from build123d import *

# Parameters (mm, degrees)
MODEL_R             = 2
MODEL_R_2           = 1.5
BOSS_EXTRUDE1_DEPTH = 6


with BuildPart() as part:
    # Model → Boss-Extrude1 (new body)
    with BuildSketch(Plane.XY):
        Polygon((136.503533409, 63.253129949), (136.50298126, 57.754435229), (123.504343338, 57.752522637), (123.503533606, 63.255740591), (110.504895018, 63.258351095), (110.504341961, 57.750609844), (97.50570415, 57.760961628), (97.504895084, 63.259656484), (84.506256496, 63.262266989), (84.505704216, 57.762267017), (71.507065628, 57.764877521), (71.508169139, 63.259656429), (71.52323132, 218.754434691), (84.52187017, 218.754434691), (84.52131789, 213.254434719), (97.51995674, 213.254434719), (97.521870105, 218.753129302), (110.520509732, 218.760870582), (110.519956675, 213.25312933), (123.518595525, 213.25312933), (123.520510463, 218.75634701), (136.519147739, 218.751823913), (136.51859559, 213.253129193), (149.517234309, 213.251823941), (149.512489722, 166.001824179), (143.512489752, 166.002426666), (143.512213612, 163.25242668), (143.511937472, 160.502426694), (149.511937442, 160.501824207), (149.50867397, 128.001824371), (143.508674, 128.002426858), (143.50839786, 125.252426872), (143.50812172, 122.502426886), (149.502172128, 122.501824996), (149.502172128, 63.251824697), align=None)
        with Locations((110.507816209, 83.257045523)):
            Circle(MODEL_R, mode=Mode.SUBTRACT)
        with Locations((110.518861547, 193.254434719)):
            Circle(MODEL_R, mode=Mode.SUBTRACT)
        with Locations((110.507264687, 138.255740731)):
            Circle(MODEL_R_2, mode=Mode.SUBTRACT)
        Polygon((119.512213733, 163.254836629), (119.512489873, 166.004836615), (125.512489843, 166.004234128), (125.511937563, 160.504234156), (119.511937593, 160.504836643), align=None, mode=Mode.SUBTRACT)
        Polygon((131.512213673, 163.253631655), (131.512489813, 166.003631641), (137.512489783, 166.003029154), (137.511937503, 160.503029181), (131.511937533, 160.503631669), align=None, mode=Mode.SUBTRACT)
        Polygon((113.511008789, 151.255439177), (113.511284929, 154.005439163), (119.511284899, 154.004836676), (119.510732619, 148.504836703), (113.510732649, 148.505439191), align=None, mode=Mode.SUBTRACT)
        Polygon((125.511008729, 151.254234202), (125.511284869, 154.004234189), (131.511284838, 154.003631701), (131.510732558, 148.503631729), (125.510732589, 148.504234216), align=None, mode=Mode.SUBTRACT)
        Polygon((137.511008668, 151.253029228), (137.511284808, 154.003029214), (143.511284778, 154.002426727), (143.510732498, 148.502426755), (137.510732528, 148.503029242), align=None, mode=Mode.SUBTRACT)
        Polygon((119.508397981, 125.254836821), (119.508674121, 128.004836807), (125.508674091, 128.00423432), (125.508121811, 122.504234347), (119.508121841, 122.504836835), align=None, mode=Mode.SUBTRACT)
        Polygon((131.50839792, 125.253631846), (131.50867406, 128.003631832), (137.50867403, 128.003029345), (137.50812175, 122.503029373), (131.50812178, 122.50363186), align=None, mode=Mode.SUBTRACT)
        Polygon((125.507192976, 113.254234394), (125.507469116, 116.00423438), (131.507469086, 116.003631893), (131.506916806, 110.503631921), (125.506916836, 110.504234408), align=None, mode=Mode.SUBTRACT)
        Polygon((137.507192916, 113.253029419), (137.507469056, 116.003029406), (143.507469025, 116.002426918), (143.506916745, 110.502426946), (137.506916776, 110.503029433), align=None, mode=Mode.SUBTRACT)
    extrude(amount=BOSS_EXTRUDE1_DEPTH)


solid = part.part
Build history of the part. All positions in model axes, mm. Round coordinates to 2 decimals unless told otherwise and drop trailing zeros. Write each loop counter-clockwise with the first axis right and the second up, starting at its lowest first coordinate (ties: lowest second). Pieces come first, ordered by that corner, then holes. Notation, with made-up numbers: M 86,-13 L 134,-13 A30 cw 134,18 Z; hole C -34.5,-29.75 d8. An arc over 180 degrees is marked long. Answer as a JSON object with one key per item and string values. Group by question number.
(1) Drill centre lines: L1, parallel to Y at x = 135, z = 0.4; L2, parallel to Y at x = 128, z = 4.8; L3, parallel to X at y = 113, z = 4.2. Where is each one in solid material? Low to high.
(2) Cut at D-D (z = 1.85). Give the number of separate pieces and of enclosed holes in the cut face, and give its area (3 significant figures).
(3) Cut at C-C (y = 125.5). Give the cut face in (x, z), and give its area (3 significant figures).
(4) Cut at A-A (x = 133). Give the cut face in (y, z).
(5) Flat gauge pins, fed straight in: pin 1 (1.8 mm diameter, centred on x = 123, z = 2, fed in from +Y); pin 2 (2.5 mm diameter, centred on y = 162.5, z = 3, fed in from +X); pin 3 (1.8 mm diameter, centred on x = 119, z = 2.5, fed in from +Y). Where does each tip first touch, or does it go through?
(6) Mould opens along Y. For faces 1 (the cylindrical face through (111.199, 136.925, 2.958)), 2 (the flat face through (78, 218.754, 3)), 3 (the cylindrical face through (112.427, 193.855, 2.958)) say: pulls with the +Y half, pulls with the -Y half, needs draft (parallel to the pull), parting line crosses it, or undercut.
(7) Cut at B-B (y = 151.5). Give the cut face in (x, z).
Responses:
{
 "1": {"L1": "y = 57.75 to 122.5, 128 to 160.5, 166 to 218.75", "L2": "y = 57.75 to 110.5, 116 to 148.5, 154 to 218.75", "L3": "x = 71.51 to 125.51, 131.51 to 137.51, 143.51 to 149.5"},
 "2": {"separate pieces": "1", "enclosed holes": "12", "area": "11,700 mm2"},
 "3": {"outline": "M 71.51,0 L 119.51,0 L 119.51,6 L 71.51,6 Z; M 125.51,0 L 131.51,0 L 131.51,6 L 125.51,6 Z; M 137.51,0 L 143.51,0 L 143.51,6 L 137.51,6 Z", "area": "360 mm2"},
 "4": {"outline": "M 57.75,0 L 122.5,0 L 122.5,6 L 57.75,6 Z; M 128,0 L 160.5,0 L 160.5,6 L 128,6 Z; M 166,0 L 218.75,0 L 218.75,6 L 166,6 Z"},
 "5": {"pin 1": "stops at y = 218.76", "pin 2": "stops at x = 143.51", "pin 3": "stops at y = 213.25"},
 "6": {"face 1": "undercut", "face 2": "pulls with the +Y half", "face 3": "undercut"},
 "7": {"outline": "M 71.52,0 L 113.51,0 L 113.51,6 L 71.52,6 Z; M 119.51,0 L 125.51,0 L 125.51,6 L 119.51,6 Z; M 131.51,0 L 137.51,0 L 137.51,6 L 131.51,6 Z; M 143.51,0 L 149.51,0 L 149.51,6 L 143.51,6 Z"}
}
